The listing builds one solid part. Answer for the finished solid, in the listing's coordinates (mm). A direction names the side the tool comes from. Give positions to 0.01 mm unless a question says otherwise; leave off trailing zeros. Write each loop counter-clockwise with the first axis right and the second up, starting at its lowest first coordinate (ties: lowest second). Pieces come first, ordered by that corner, then holes. Notation, with made-up numbers: (14.25, 20.25) - (26.25, 20.25) arc R8 ccw to (26.25, 31.25) - close; hole circle Ø1 at (-13.5, 14). An arc over 180 degrees is marked (long way). Answer as CSV lines item,"result". Start each with the question number.
(1) Find section D-D (z = 1.5). Write down the section's boundary in (x, y), then the cut area to 3 significant figures.
(2) Find section A-A (z = 0). Write down the section's boundary in (x, y), then the cut area to 3 significant figures.
(3) For a pull along X with two mould halves and no side action, classify faces 1 (the face through (0, 8, 0)), 2 (the face through (-5.734, 0.986, 0.421)), 3 (the face through (7.766, 0.986, 0.421)), 4 (the face through (11.25, 0.99, -0.1)) as pulls with the +X half, pulls with the -X half, needs draft (parallel to the pull), parting line crosses it, or undercut.
(4) Straight lines are drawn through the part: probe 1 along X at (y, z) = (1.55, 0); probe 2 along Z at (x, y) = (-6.75, 1.4); probe 3 along Y at (x, z) = (8.5, -4). For each, find the intervals that lie inside material, in ascending order.
(5) Find section B-B (y = 1.75). Write down the section's boundary in (x, z), then the cut area to 3 significant figures.
(6) Find section C-C (x = 0). Write down the section's boundary in (y, z).
(7) Each of these flat-tipped pins is pushed along its axis until it touches: pin 1 Ø2.5 at (x, z) = (6.75, 0) entering from -Y; pin 2 Ø4 at (y, z) = (6.5, 1) entering from +X; pin 3 Ø2 at (y, z) = (2, 1.5) entering from -X. Where does it stop, or does it pass through?
(8) For faces 5 (the face through (0, 1, -4.5)), 6 (the face through (-3.746, 4.958, 0.165)), determine the directions among +Z, -Z, +X, -X, +Y, -Y from which every point of the face is accessible in a straight line to the end or side of a thin tool.
from build123d import *

# Parameters (mm, degrees)
SKETCH1_R           = 1.1
SKETCH1_R_2         = 3.75
BOSS_EXTRUDE3_DEPTH = 2
SKETCH3_R           = 3.75
BOSS_EXTRUDE4_DEPTH = 8


with BuildPart() as part:
    # Sketch1 → Boss-Extrude3 (new body)
    with BuildSketch(Plane(origin=(0, 0, 0), x_dir=(1, 0, 0), z_dir=(0, 1, 0))):
        with BuildLine():
            Line((-6.75, 4.499502967), (6.75, 4.499502967))
            ThreePointArc((6.75, 4.499502967), (11.249502967, 0), (6.75, -4.499502967))
            Line((6.75, -4.499502967), (-6.75, -4.499502967))
            ThreePointArc((-6.75, -4.499502967), (-11.249502967, 0), (-6.75, 4.499502967))
        make_face()
        with Locations((-6.75, 0)):
            Circle(SKETCH1_R, mode=Mode.SUBTRACT)
        with Locations((6.75, 0)):
            Circle(SKETCH1_R, mode=Mode.SUBTRACT)
        Circle(SKETCH1_R_2, mode=Mode.SUBTRACT)
    extrude(amount=BOSS_EXTRUDE3_DEPTH)

    # Sketch3 → Boss-Extrude4 (add)
    with BuildSketch(Plane.XZ):
        Circle(SKETCH3_R)
    extrude(amount=-BOSS_EXTRUDE4_DEPTH)


solid = part.part
Result set:
1,outline,"(-10.99, 0) - (10.99, 0) - (10.99, 2) - (3.44, 2) - (3.44, 8) - (-3.44, 8) - (-3.44, 2) - (-10.99, 2) - close"
1,area,"85.2 mm^2"
2,outline,"(-11.25, 0) - (-7.85, 0) - (-7.85, 2) - (-11.25, 2) - close; (-5.65, 0) - (5.65, 0) - (5.65, 2) - (3.75, 2) - (3.75, 8) - (-3.75, 8) - (-3.75, 2) - (-5.65, 2) - close; (7.85, 0) - (11.25, 0) - (11.25, 2) - (7.85, 2) - close"
2,area,"81.2 mm^2"
3,face 1,"needs draft"
3,face 2,"undercut"
3,face 3,"undercut"
3,face 4,"pulls with the +X half"
4,probe 1,"-11.25 to -7.85, -5.65 to 5.65, 7.85 to 11.25"
4,probe 2,"-4.5 to -1.1, 1.1 to 4.5"
4,probe 3,"0 to 2"
5,outline,"(-6.75, -4.5) - (6.75, -4.5) arc R4.5 ccw to (6.75, 4.5) - (-6.75, 4.5) arc R4.5 ccw to start; hole circle Ø2.2 at (-6.75, 0); hole circle Ø2.2 at (6.75, 0)"
5,area,"177 mm^2"
6,outline,"(0, -4.5) - (2, -4.5) - (2, -3.75) - (8, -3.75) - (8, 3.75) - (2, 3.75) - (2, 4.5) - (0, 4.5) - close"
7,pin 1,"y = 0"
7,pin 2,"x = 3.75"
7,pin 3,"x = -11.22"
8,face 5,"-Z, +X, -X, +Y, -Y"
8,face 6,"+Y"
